Work out the finished part from the listing and answer in its coordinate system (mm). Face numbers are marked on the shaded views. Give positions to 0.01 mm unless a question says otherwise; leave off trailing zeros. Loops run counter-clockwise (first coordinate to the right, second up) from the corner with the lowest first, then second, coordinate; pieces in that order, holes last. Notation, with made-up numbers: (73.5, 63) - (101.5, 63) arc R31 ccw to (101.5, 87) - close; hole circle Ø11 at (34.5, 47). An arc over 180 degrees is marked (long way). One line per question, with ' | ' between items.
from build123d import *

# Parameters (mm, degrees)
F0_W      = 145
F0_H      = 80
F1_DEPTH  = 2
F2_W      = 141
F2_H      = 76
F3_DEPTH  = 1
F5_DEPTH  = 25
F6_R      = 1
F7_DEPTH  = 25
F8_W      = 1
F8_H      = 2
F9_DEPTH  = 200
F10_R     = 1
F11_DEPTH = 80
F12_R     = 0.5
F13_DEPTH = 300
F15_DEPTH = 1.5


with BuildPart() as f1:
    # F0 (on Front) → F1 (new body)
    with BuildSketch(Plane.XZ):
        Rectangle(F0_W, F0_H)
    extrude(amount=F1_DEPTH)

    # F2 (on face) → F3 (join)
    with BuildSketch(Plane(origin=(0, 0, 0), x_dir=(-1, 0, 0), z_dir=(0, 1, 0))):
        Rectangle(F2_W, F2_H)
    extrude(amount=F3_DEPTH)

    # F4 (on face) → F5 (cut)
    with BuildSketch(Plane.XZ.offset(2)):
        with BuildLine():
            Line((3, -4.5), (3, 4.5))
            ThreePointArc((3, 4.5), (0, 7.5), (-3, 4.5))
            Line((-3, 4.5), (-3, -4.5))
            ThreePointArc((-3, -4.5), (0, -7.5), (3, -4.5))
        make_face()
    extrude(amount=-F5_DEPTH, mode=Mode.SUBTRACT)

    # F6 (on face) → F7 (cut)
    with BuildSketch(Plane.XZ.offset(2)):
        with Locations((-6.5, 16.5)):
            Circle(F6_R)
        with Locations((6.5, 16.5)):
            Circle(F6_R)
        with Locations((6.5, -7.5)):
            Circle(F6_R)
        with Locations((-6.5, -7.5)):
            Circle(F6_R)
        with Locations((-6.5, 4.5)):
            Circle(F6_R)
        with Locations((6.5, 4.5)):
            Circle(F6_R)
    extrude(amount=-F7_DEPTH, mode=Mode.SUBTRACT)

    # F8 (on face) → F9 (cut)
    with BuildSketch(Plane.XY.offset(40)):
        with Locations((72, -1)):
            Rectangle(F8_W, F8_H)
    extrude(amount=-F9_DEPTH, mode=Mode.SUBTRACT)

    # F10 (on face) → F11 (join)
    with BuildSketch(Plane.XY.offset(40)):
        with Locations((71.5, -1)):
            Circle(F10_R)
    extrude(amount=-F11_DEPTH)

    # F12 (on face) → F13 (cut)
    with BuildSketch(Plane.XY.offset(40)):
        with Locations((71.5, -1)):
            Circle(F12_R)
    extrude(amount=-F13_DEPTH, mode=Mode.SUBTRACT)

    # F14 (on face) → F15 (cut)
    with BuildSketch(Plane(origin=(0, 1, 0), x_dir=(-1, 0, 0), z_dir=(0, 1, 0))):
        with BuildLine():
            Line((-4.5, -4.5), (-3, -4.5))
            Line((-3, -4.5), (3, -4.5))
            Line((3, -4.5), (4.5, -4.5))
            Line((4.5, -4.5), (4.5, 17.037205))
            ThreePointArc((4.5, 17.037205), (0, 21.537205), (-4.5, 17.037205))
            Line((-4.5, 17.037205), (-4.5, -4.5))
        make_face()
    extrude(amount=-F15_DEPTH, mode=Mode.SUBTRACT)


solid = f1.part
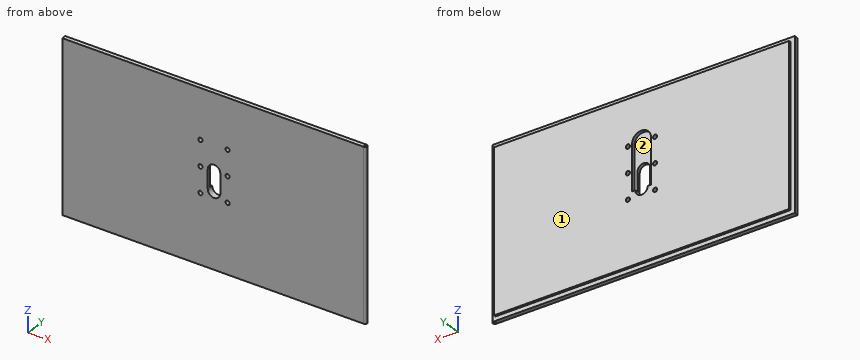
1. Consider L1, parallel to Z at x = 6.5, y = -0.65; L2, parallel to X at y = -1.15, z = 35; L3, parallel to X at y = 0.75, z = -22. Determine where each line is inside the solid, lowest interval first.
Evaluation:
L1: -40 to -8.5, -6.5 to 3.5, 5.5 to 15.5, 17.5 to 40 | L2: -72.5 to 71.02, 71.98 to 72.49 | L3: -70.5 to 70.5
2. Find section C-C on x = 51. Write down the section's boundary in (y, z), then the cut area to 3 significant figures.
Evaluation:
outline: (-2, -40) - (0, -40) - (0, -38) - (1, -38) - (1, 38) - (0, 38) - (0, 40) - (-2, 40) - close | area: 236 mm2
3. Find section B-B on x = 0. Write down the section's boundary in (y, z), then the cut area to 3 significant figures.
Evaluation:
outline: (-2, -40) - (0, -40) - (0, -38) - (1, -38) - (1, -7.5) - (-2, -7.5) - close; (-2, 7.5) - (-0.5, 7.5) - (-0.5, 21.54) - (1, 21.54) - (1, 38) - (0, 38) - (0, 40) - (-2, 40) - close | area: 170 mm2
4. Flat-ended cylindrical pins translate along their axes: pin 1 (0.5 mm diameter, centred on y = 0.5, z = -10.5, fed in from +X); pin 2 (1.2 mm diameter, centred on x = -6.5, z = -7.5, fed in from +Y); pin 3 (0.8 mm diameter, centred on x = 3.5, y = 0.5, fed in from +Z). Find the tip coordinate at first contact, or state that the pin passes through.
Evaluation:
pin 1: x = 70.5 | pin 2: through | pin 3: z = 38
5. Determine the mould class of the marked faces 1 and 2 for opening direction Z: +Z half, -Z half, draft (parallel to the pull), parting line (faces both ways), or undercut.
Evaluation:
face 1: draft | face 2: undercut
6. Find section A-A on y = -1. State how many separate pieces and enclosed holes the cut face has, then the cut area to 3 significant figures.
Evaluation:
separate pieces: 2 | enclosed holes: 7 | area: 11,400 mm2
